Input: dimensioned drawing with shaded views. Units: mm. Origin: part minimum x, y, z. Coordinates: 2 decimals unless noted, no trailing zeros. Order: outer loops, then holes, each group sorted by start corner. A loop starts at its lowest first (then second) coordinate and runs counter-clockwise, first axis right, second up. Notation, with made-up numbers: (35.25, 16) -> (91.25, 16) arc R32 ccw to (91.25, 54) -> close; hole circle Ø11 at (-6.75, -1.5). An arc over 180 degrees is marked (long way). Answer in a Markdown table with one row per item. Add a question column.
1) Section query A-A on z = 8. Return the cut outline in (x, y), then the cut area to 3 significant figures.
2) Contact query for flat-ended pins moving along their axis: P1, Ø2, axis at y = 4, z = 1.5, coming from the -X side; P2, Ø1, axis at x = 3, z = 4, coming from the +Y side. Output: stop coordinate, or through.
3) Ray query, line 1 (X direction, y = 2.65, z = 3.5) (1 decimal); line 2 (Y direction, x = 2.15, z = 6.25); line 3 (X direction, y = 1.4, z = 2). Return the intervals inside material, ascending. Write a range as from..to.
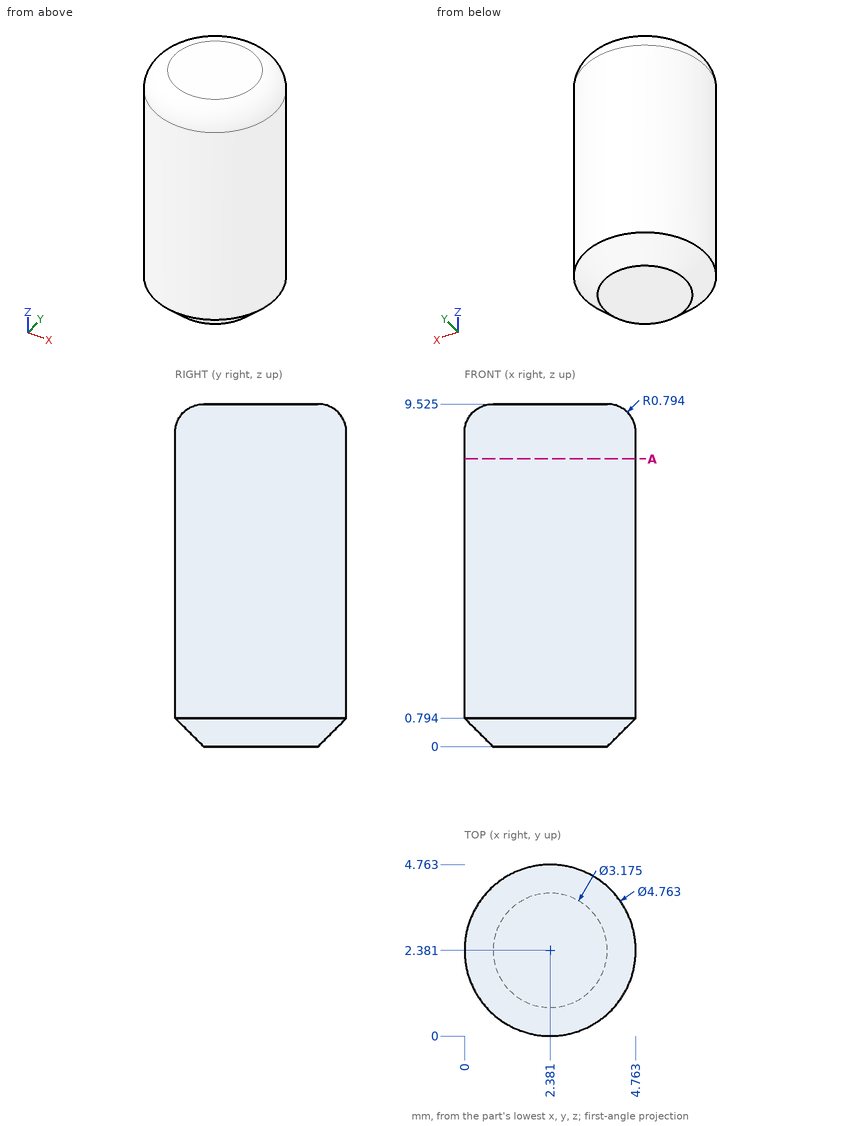
Result:
| question | item | result |
|---|---|---|
| 1 | outline | circle Ø4.76 at (2.38, 2.38) |
| 1 | area | 17.8 mm2 |
| 2 | P1 | x = 0.08 |
| 2 | P2 | y = 4.76 |
| 3 | line 1 | 0..4.7 |
| 3 | line 2 | 0.01..4.75 |
| 3 | line 3 | 0.21..4.55 |
